Autodesk Fusion 360 part; units mm, degrees
sketch "Sketch1" plane through (0, 0, 0) normal (0, 1, 0) x (1, 0, 0)
  line L0 (-100, -1.1649) -> (40, -1.1649)
  line L1 (40, -1.1649) -> (40, -55.1649)
  line L2 (40, -55.1649) -> (22, -55.1649)
  line L3 (-100, -1.1649) -> (-100, -29.1649)
  line L4 (22, -55.1649) -> (22, -29.1649)
  circle A0 centre (-50, -66.1649) radius 25
  circle A1 centre (-50, -66.1649) radius 14
  line L5 (-25, -66.1649) -> (-25, -29.1649)
  line L6 (-75, -66.1649) -> (-75, -29.1649)
  line L7 (22, -29.1649) -> (-25, -29.1649)
  line L8 (-75, -29.1649) -> (-100, -29.1649)
  line L9 (22, -29.1649) -> (40, -29.1649)
  line L10 (-100, -1.1649) -> (-117.3228, -1.1649)
  line L11 (-117.3228, -1.1649) -> (-117.3228, -16.1649)
  line L12 (-117.3228, -16.1649) -> (-100, -16.1649)
  line L13 (-100, -16.1649) -> (40, -16.1649)
  line L14 (-75, -29.1649) -> (-75, -1.1649)
  line L15 (-25, -29.1649) -> (-25, -1.1649)
  line L16 (22, -29.1649) -> (22, -1.1649)
  dimension "d1" = 140
  dimension "d2" = 54
  dimension "d3" = 18
  dimension "d6" = 28
  dimension "d7" = 50
  dimension "d8" = 28
  dimension "d9" = 65
  dimension "d10" = 90
  dimension "d11" = 15
extrude "Extrude1" add sketch "Sketch1" along normal blind 82 contours L0 L3 L13 L14 | L3 L10 L11 L12 | L0 L13 L14 L15 | L0 L13 L15 L16 | L0 L1 L13 L16 | L1 L9 L13 L16 | L1 L2 L4 L9
extrude "Extrude2" add sketch "Sketch1" along normal blind 12 contours L3 L8 L13 L14 | L7 L13 L15 L16
extrude "Extrude3" add sketch "Sketch1" along normal blind 22 contours A0 L5 L6 L13 L14 L15 | A0
ref_plane "WorkPlane1" through (-38.6614, 41, 28.1649) normal (0, 1, 0) x (0, 0, 1)
mirror "Mirror1" about plane through (-38.6614, 41, 28.1649) normal (0, 1, 0) of "Extrude3"
mirror "Mirror2" about plane through (-38.6614, 41, 28.1649) normal (0, 1, 0) of "Extrude2"
sketch "Sketch2" plane through (40, 0, 0) normal (1, 0, 0) x (0, 1, 0)
  line L0 (0, 55.1649) -> (0, 1.1649)
  line L1 (0, 1.1649) -> (82, 1.1649)
  line L2 (82, 1.1649) -> (82, 55.1649)
  line L3 (82, 55.1649) -> (0, 55.1649)
  arc A0 (28.5, 55.1649) -> (53.5, 55.1649) centre (41, 55.1649) ccw
  arc A1 (21.8899, 55.1649) -> (60.1101, 55.1649) centre (41, 55.1649) ccw
  dimension "d22" = 25
extrude "Extrude4" add sketch "Sketch2" against normal blind 28 contours L3 A0 A1
extrude "Extrude5" cut sketch "Sketch2" against normal blind 28 contours L3 A0
sketch "Sketch3" plane through (0, 0, 16.1649) normal (0, 0, 1) x (-1, 0, 0)
  line L0 (-22, -70) -> (25, -70)
  line L1 (25, -70) -> (25, -60)
  line L2 (25, -60) -> (75, -60)
  line L3 (75, -60) -> (75, -70)
  line L4 (75, -70) -> (100, -70)
  line L5 (100, -70) -> (100, -82)
  line L6 (100, -82) -> (117.3228, -82)
  line L7 (117.3228, -82) -> (117.3228, 0)
  line L8 (117.3228, 0) -> (100, 0)
  line L9 (100, 0) -> (100, -12)
  line L10 (100, -12) -> (75, -12)
  line L11 (75, -12) -> (75, -22)
  line L12 (75, -22) -> (25, -22)
  line L13 (25, -22) -> (25, -12)
  line L14 (25, -12) -> (-22, -12)
  line L15 (-22, -12) -> (-22, -70)
  line L16 (100, -12) -> (100, -70) construction
  line L17 (117.3228, -41) -> (75, -41) construction
  circle A0 centre (100, -41) radius 11
  circle A1 centre (100, -41) radius 18
  line L18 (100, -12) -> (100, -70)
  dimension "d27" = 22
  dimension "d28" = 36
extrude "Extrude6" cut sketch "Sketch3" against normal blind 30 contours L5 L6 L7 A1 L18 | L7 L8 L9 A1 L18
extrude "Extrude7" cut sketch "Sketch3" against normal blind 25 contours A0 L18 | A0 L18
equation "d28 = 18 mm + 18 mm"
For this review, take the finished solid that the model builds, in its own axes (mm). A direction names the side the tool comes from. Round coordinates to 2 decimals unless told otherwise and drop trailing zeros. Write each loop counter-clockwise with the first axis right and the second up, starting at its lowest first coordinate (ties: lowest second). Pieces come first, ordered by that corner, then holes. Notation, with made-up numbers: (-2, -4.5) -> (7, -4.5) arc R30 cw to (7, 30.5) -> close; hole circle Ø2 at (75, 54.25). An arc over 180 degrees is marked (long way). Use one line per item in the form item = value.
1) Take a section at C-C, the plane y = 67. Write out the cut boundary in (x, z).
Found:
outline = (-100, 1.16) -> (40, 1.16) -> (40, 55.16) -> (22, 55.16) -> (22, 16.16) -> (-25, 16.16) -> (-25, 66.16) arc R25 ccw to (-75, 66.16) -> (-75, 16.16) -> (-100, 16.16) -> close; hole circle Ø28 at (-50, 66.16)
2) Take a section at A-A, the plane y = 41. Write out the cut boundary in (x, z).
Found:
outline = (-117.32, 1.16) -> (-111, 1.16) -> (-111, 16.16) -> (-117.32, 16.16) -> close; (-89, 1.16) -> (40, 1.16) -> (40, 42.66) -> (12, 42.66) -> (12, 36.05) -> (22, 36.05) -> (22, 16.16) -> (-89, 16.16) -> close
3) To check wall thickness, follow L1, parallel to Y at x = -32.5, z = 68; L2, parallel to X at y = 41, z = 14.5; L3, parallel to Z at x = -50, y = 15. State the ranges of each line that lie inside material, in increasing order. Write a range as from..to.
Found:
L1 = 0..22, 60..82
L2 = -117.32..-111, -89..40
L3 = 1.16..52.16, 80.16..91.16
4) Mouldability with a two-part tool opening along Y and no side actions: class faces 1 (the cylindrical face through (-110.992, 26.746, 8.77)), 2 (the flat face through (29, 68, 55.165)), 3 (the cylindrical face through (-110.73, 55.45, 8.77)), 4 (the flat face through (-50, 60, 45)) as +Y half, -Y half, draft (parallel to the pull), parting line (faces both ways), or undercut.
Found:
face_1 = -Y half
face_2 = draft
face_3 = +Y half
face_4 = undercut
5) Tool access review of faces 5 (the flat face through (-100, 9, 12)), 6 (the flat face through (-88, 12, 23)), 7 (the flat face through (-2, 12, 23)): name each direction out of +Z, -Z, +X, -X, +Y, -Y from which nothing blocks a thin tool from reaching the whole face with its end or side.
Found:
face_5 = +Z, -Z, -X, -Y
face_6 = +Z, -X
face_7 = +Z
6) Take a section at D-D, the plane z = 60. Write out the cut boundary in (x, y).
Found:
outline = (-75, 0) -> (-62.57, 0) -> (-62.57, 22) -> (-75, 22) -> close; (-75, 60) -> (-62.57, 60) -> (-62.57, 82) -> (-75, 82) -> close; (-37.43, 0) -> (-25, 0) -> (-25, 22) -> (-37.43, 22) -> close; (-37.43, 60) -> (-25, 60) -> (-25, 82) -> (-37.43, 82) -> close
7) Clearance check with flat-ended pins moving along their axes: pin 1 (3.5 mm diameter, centred on x = 3.5, y = 9, fed in from +Z); pin 2 (17.5 mm diameter, centred on y = 12, z = 41, fed in from -X); pin 3 (20 mm diameter, centred on x = -100, y = 41, fed in from -Z); pin 4 (12 mm diameter, centred on y = 12, z = 18, fed in from -X). State where each tip first meets the part, or that it passes through.
Found:
pin_1 = 29.16
pin_2 = -75
pin_3 = through
pin_4 = -100
8) Take a section at B-B, the plane x = -50. Write out the cut boundary in (y, z), and give its area (3 significant figures).
Found:
outline = (0, 1.16) -> (82, 1.16) -> (82, 52.16) -> (60, 52.16) -> (60, 16.16) -> (22, 16.16) -> (22, 52.16) -> (0, 52.16) -> close; (0, 80.16) -> (22, 80.16) -> (22, 91.16) -> (0, 91.16) -> close; (60, 80.16) -> (82, 80.16) -> (82, 91.16) -> (60, 91.16) -> close
area = 3,300 mm2
